Design review of the part built by this model. Coordinates are the model's own, in mm. A direction names the side the tool comes from. Round coordinates to 2 decimals unless told otherwise and drop trailing zeros. Order: outer loops, then holes, each group sorted by start corner. A loop starts at its lowest first (then second) coordinate and runs counter-clockwise, first axis right, second up. Notation, with made-up numbers: (68, 63.25) - (78, 63.25) arc R18 cw to (78, 96.25) - close; hole circle Ø11 at (-15.5, -33). An arc over 180 degrees is marked (long way). Write item = value, one per line.
from build123d import *

# Parameters (mm, degrees)
SKETCH2_W               = 50
SKETCH2_H               = 250
BOSS_EXTRUDE1_DEPTH     = 20
CUT_EXTRUDE1_DEPTH      = 256.734237051
CUT_EXTRUDE1_DEPTH_BACK = 256.734237051
SKETCH3_OUTSIDE_W       = 303.146
SKETCH3_OUTSIDE_H       = 73.146
CUT_EXTRUDE2_START      = -10
CUT_EXTRUDE2_DEPTH      = 30


with BuildPart() as part:
    # Sketch2 → Boss-Extrude1 (new body)
    with BuildSketch(Plane(origin=(0, 0, 0), x_dir=(1, 0, 0), z_dir=(0, 1, 0))):
        with Locations((25, 125)):
            Rectangle(SKETCH2_W, SKETCH2_H)
    extrude(amount=BOSS_EXTRUDE1_DEPTH)

    # Sketch3 outside → Cut-Extrude1 (cut, two sides: drawn at the far end of the back side and taken through both)
    with BuildSketch(Plane(origin=(50, 0, 0), x_dir=(0, 0, -1), z_dir=(1, 0, 0)).offset(-CUT_EXTRUDE1_DEPTH_BACK)):
        with Locations((125, 10)):
            Rectangle(SKETCH3_OUTSIDE_W, SKETCH3_OUTSIDE_H)
        Polygon((0, 0), (11.547005384, 20), (250, 20), (238.452994616, 0), align=None, mode=Mode.SUBTRACT)
    extrude(amount=CUT_EXTRUDE1_DEPTH + CUT_EXTRUDE1_DEPTH_BACK, mode=Mode.SUBTRACT)

    # Sketch4 → Cut-Extrude2 (cut)
    with BuildSketch(Plane(origin=(50, 0, 0), x_dir=(0, 0, -1), z_dir=(1, 0, 0)).offset(CUT_EXTRUDE2_START)):
        Polygon((11.547005384, 20), (250, 20), (241.339745962, 5), (2.886751346, 5), align=None)
    extrude(amount=-CUT_EXTRUDE2_DEPTH, mode=Mode.SUBTRACT)


solid = part.part
Item 1: For faces 1 (the face through (5, 20, -132)), 2 (the face through (40, 13, -128)), list the 3-axis set-ups (+Z, -Z, +X, -X, +Y, -Y) from which the entire face can be reached by the end or side of a thin tool; tool diameter is ignored.
Data:
face_1 = +Z, -Z, +X, -X, +Y
face_2 = +Z, -Z, +Y
Item 2: For line 1 along X through (y, z) = (13, -153.5); line 2 along Y through (x, z) = (15, -196); line 3 along Z through (x, y) = (29, 3), list the stretches that pass through material, from the lowest coordinate up. Write a range as [from, to].
Data:
line_1 = [0, 10], [40, 50]
line_2 = [0, 5]
line_3 = [-240.19, -1.73]
Item 3: Insertion check: P1, Ø2, axis at x = 20, z = -156, coming from the +Y side; P2, Ø1.5, axis at x = 6.5, y = 17, coming from the -Z side. Each pin has a flat end and moves straight along its axis. Give the tip position at first contact, or say it passes through.
Data:
P1 = 5
P2 = -248.7
Item 4: Take a section at B-B, the plane z = -124.5. State the section outline as (x, y) points.
Data:
outline = (0, 0) - (50, 0) - (50, 20) - (40, 20) - (40, 5) - (10, 5) - (10, 20) - (0, 20) - close
Item 5: Take a section at A-A, the plane y = 13.5. State the section outline as (x, z) points, and give its area (3 significant figures).
Data:
outline = (0, -246.25) - (10, -246.25) - (10, -7.79) - (0, -7.79) - close; (40, -246.25) - (50, -246.25) - (50, -7.79) - (40, -7.79) - close
area = 4,770 mm2
Item 6: The part is to be moulded in two halves that separate along X. For faces 3 (the face through (24.65, 3.19, -1.84)), 4 (the face through (10, 13, -128)), 5 (the face through (50, 10, -123)), say which applies: +X half, -X half, draft (parallel to the pull), parting line (faces both ways), or undercut.
Data:
face_3 = draft
face_4 = undercut
face_5 = +X half
Item 7: Take a section at D-D, the plane x = 44.5. State the section outline as (y, z) points, and give its area (3 significant figures).
Data:
outline = (0, -238.45) - (20, -250) - (20, -11.55) - (0, 0) - close
area = 4,770 mm2
Item 8: Take a section at C-C, the plane x = 22.5. State the section outline as (y, z) points, and give its area (3 significant figures).
Data:
outline = (0, -238.45) - (5, -241.34) - (5, -2.89) - (0, 0) - close
area = 1,190 mm2
